CAD build for the part. Positions are in the model's coordinates, mm. Round coordinates to 2 decimals unless told otherwise and drop trailing zeros. Loops run counter-clockwise (first coordinate to the right, second up) from the corner with the lowest first, then second, coordinate; pieces in that order, holes last. Notation, with made-up numbers: M 13,77 L 58,77 A29 cw 58,115 Z; hole C -19,28 d9. An arc over 180 degrees is marked long. One line per item, written item: value. Start each with the question number.
Autodesk Inventor part; units mm, degrees
ref_plane "YZ Plane" through (0, 0, 0) normal (1, 0, 0) x (0, 1, 0)
ref_plane "XZ Plane" through (0, 0, 0) normal (0, 1, 0) x (-1, 0, 0)
ref_plane "XY Plane" through (0, 0, 0) normal (0, 0, 1) x (1, 0, 0)
sketch "스케치1" plane through (0, 0, 0) normal (0, 0, 1) x (1, 0, 0)
  line L0 (-0.0808, 29.1134) -> (-0.0808, -34.3055)
  line L1 (-44.0255, 0.0549) -> (53.8558, 0.0549)
  line L2 (-35.8687, -7.9451) -> (-35.8687, -23.9451)
  line L3 (-35.8687, -23.9451) -> (-35.8687, 0.0549)
  line L4 (-35.8687, 8.0549) -> (-35.8687, 24.0549)
  line L5 (-35.8687, 24.0549) -> (5.7005, 0.0549)
  line L6 (-35.8687, -23.9451) -> (5.7005, 0.0549)
  arc A0 (-35.8687, -15.2849) -> (-28.3687, -19.615) centre (-30.8687, -15.2849) ccw
  arc A1 (-28.3687, 19.7248) -> (-35.8687, 15.3946) centre (-30.8687, 15.3946) ccw
  arc A2 (-35.8687, -7.9451) -> (-35.8687, 8.0549) centre (-35.8687, 0.0549) ccw
  line L7 (-15.8687, 16.9552) -> (-15.8687, -23.9451)
  arc A3 (-11.8687, 8.0549) -> (-11.8687, -7.9451) centre (-5.8687, 0.0549) ccw
  line L8 (-11.8687, 10.1985) -> (-11.8687, 8.0549)
  line L9 (-11.8687, -7.9451) -> (-11.8687, -10.0887)
  dimension "d7" = 24
  dimension "d8" = 24
  dimension "d9" = 60
  dimension "d10" = 10
  dimension "d11" = 10
  dimension "d12" = 16
  dimension "d14" = 20
sketch "스케치2" plane through (0, 0, 0) normal (0, 0, 1) x (1, 0, 0)
  point P0 (0, 0)
extrude "돌출1" add sketch "스케치1" along normal blind 10 contours L8 A3 L7 L5 | L7 L6 A0 L2 A2 L1 | L1 A2 L4 A1 L5 L7 | A3 L9 L6 L7
sketch "스케치3" plane through (0, 0, 10) normal (0, 0, 1) x (1, 0, 0)
  point P0 (0, 0)
sketch "스케치4" plane through (0, 0, 10) normal (0, 0, 1) x (1, 0, 0)
  point P0 (0, 0)
properties part number "240412_sketch3"
(1) Slice it at C-C, the plane x = -14.5. List the corners of the cut face in (y, z), and give its area (3 significant figures).
(2) Probe L1, parallel to Y at x = -34, z = 5.5; L2, parallel to Y at x = -32, z = 8.5 (3 decimals); L3, parallel to X at y = 5, z = 6.5. List the from-to ranges inside material, lowest first.
(3) Slice it at B-B, the plane z = 6.5. List the corners of the cut face in (x, y) (1 decimal).
(4) Slice it at A-A, the plane x = -32.75. List the corners of the cut face in (y, z), and give its area (3 significant figures).
(5) Flat gauge pins, fed straight in: P1, Ø5, axis at x = -18.5, z = 5, coming from the -Y side; P2, Ø6, axis at y = -3.5, z = 4, coming from the -X side; P3, Ø1.5, axis at x = -29.5, z = 6, coming from the +Y side. Where does each tip first touch, or does it go through?
(6) Mould opens along Y. For faces 1 (the cylindrical face through (-27.87, 0.23, 4.93)), 2 (the flat face through (-11.869, 9, 5)), 3 (the flat face through (-20.2, -14.9, 4.9)) say: pulls with the +Y half, pulls with the -Y half, needs draft (parallel to the pull), parting line crosses it, or undercut.
(7) Slice it at D-D, the plane y = -13. List the corners of the cut face in (x, z).
Check result:
1. outline: M -11.61,0 L -4.99,0 L -4.99,10 L -11.61,10 Z; M 5.1,0 L 11.72,0 L 11.72,10 L 5.1,10 Z
1. area: 132 mm^2
2. L1: y = -19.18 to -7.72, 7.83 to 19.29
2. L2: y = -20.155 to -6.947, 7.057 to 20.265
2. L3: x = -29.58 to -14.56
3. outline: M -35.9,-15.3 A5 ccw -28.4,-19.6 L -11.9,-10.1 L -11.9,-7.9 A10 cw -11.9,8.1 L -11.9,10.2 L -28.4,19.7 A5 ccw -35.9,15.4 L -35.9,8.1 A8 cw -35.9,-7.9 Z
4. outline: M -19.92,0 L -7.31,0 L -7.31,10 L -19.92,10 Z; M 7.42,0 L 20.03,0 L 20.03,10 L 7.42,10 Z
4. area: 252 mm^2
5. P1: stops at y = -15.36
5. P2: stops at x = -31.28
5. P3: stops at y = 20.36
6. face 1: undercut
6. face 2: needs draft
6. face 3: pulls with the -Y half
7. outline: M -35.87,0 L -16.91,0 L -16.91,10 L -35.87,10 Z
